```python
from build123d import *

# Parameters (mm, degrees)
SKETCH1_R           = 45
SKETCH1_R_2         = 20
BOSS_EXTRUDE1_DEPTH = 15
SKETCH2_R           = 7.5
CUT_EXTRUDE1_DEPTH  = 15


with BuildPart() as part:
    # Sketch1 → Boss-Extrude1 (new body)
    with BuildSketch(Plane.XY):
        Circle(SKETCH1_R)
        Circle(SKETCH1_R_2, mode=Mode.SUBTRACT)
    extrude(amount=BOSS_EXTRUDE1_DEPTH)

    # Sketch2 → Cut-Extrude1 (cut)
    with BuildSketch(Plane.XY.offset(15)):
        with Locations((0, 45)):
            Circle(SKETCH2_R)
        with Locations((17.220754456, 41.574578963)):
            Circle(SKETCH2_R)
        with Locations((31.819805153, 31.819805153)):
            Circle(SKETCH2_R)
        with Locations((41.574578963, 17.220754456)):
            Circle(SKETCH2_R)
        with Locations((45, 0)):
            Circle(SKETCH2_R)
        with Locations((41.574578963, -17.220754456)):
            Circle(SKETCH2_R)
        with Locations((31.819805153, -31.819805153)):
            Circle(SKETCH2_R)
        with Locations((17.220754456, -41.574578963)):
            Circle(SKETCH2_R)
        with Locations((0, -45)):
            Circle(SKETCH2_R)
        with Locations((-17.220754456, -41.574578963)):
            Circle(SKETCH2_R)
        with Locations((-31.819805153, -31.819805153)):
            Circle(SKETCH2_R)
        with Locations((-41.574578963, -17.220754456)):
            Circle(SKETCH2_R)
        with Locations((-45, 0)):
            Circle(SKETCH2_R)
        with Locations((-41.574578963, 17.220754456)):
            Circle(SKETCH2_R)
        with Locations((-31.819805153, 31.819805153)):
            Circle(SKETCH2_R)
        with Locations((-17.220754456, 41.574578963)):
            Circle(SKETCH2_R)
    extrude(amount=-CUT_EXTRUDE1_DEPTH, mode=Mode.SUBTRACT)


solid = part.part
```
Can you work these out from the model? Positions are in its coordinate system, mm. Round coordinates to 2 decimals unless told otherwise and drop trailing zeros. Loops run counter-clockwise (first coordinate to the right, second up) from the corner with the lowest first, then second, coordinate; pieces in that order, holes last.
Item 1: Will these pins go through, and if not, where does the flat tip stop? pin 1 Ø5 at (y, z) = (0.5, 9.5) entering from -X; pin 2 Ø5 at (y, z) = (0.5, 5.5) entering from +X; pin 3 Ø1.5 at (x, y) = (-12.5, -14) entering from -Z; pin 4 Ø5 at (y, z) = (-28, 13.5) entering from -X.
Item 2: If we mould it in two halves opening along X, with no side actions, what happens to faces 1 (the cylindrical face through (-44.14, -8.76, 7.4)), 2 (the cylindrical face through (-0.16, 37.5, 7.6)), 3 (the cylindrical face through (-26.407, -26.628, 7.605)), 4 (the cylindrical face through (37.426, 24.985, 7.395))? For each: +X half, -X half, draft (parallel to the pull), parting line (faces both ways), or undercut.
Item 3: Please list where these lines run through material, in increasing order: L1, parallel to X at y = -25, z = 11; L2, parallel to Y at x = -35, z = 3.75; L3, parallel to Y at x = -36.5, z = 7.25.
Item 4: Suppose I cut it at A-A, the plane x = 0. Write out the boundary of the cut face in (y, z).
Reported:
1. pin 1: stops at x = -38.13
1. pin 2: stops at x = 38.13
1. pin 3: passes through
1. pin 4: stops at x = -37.08
2. face 1: -X half
2. face 2: undercut
2. face 3: undercut
2. face 4: +X half
3. L1: x = -37.42 to -34.94, -28.7 to 28.7, 34.94 to 37.42
3. L2: y = -25.03 to -20.83, -13.61 to 13.61, 20.83 to 25.03
3. L3: y = -25.96 to -22.74, -11.7 to 11.7, 22.74 to 25.96
4. outline: (-37.5, 0) - (-20, 0) - (-20, 15) - (-37.5, 15) - close; (20, 0) - (37.5, 0) - (37.5, 15) - (20, 15) - close
